Work out the finished part from the listing and answer in its coordinate system (mm). Give positions to 0.01 mm unless a question says otherwise; leave off trailing zeros. Loops run counter-clockwise (first coordinate to the right, second up) from the corner with the lowest first, then second, coordinate; pieces in that order, holes last. Notation, with made-up numbers: (69, 65.25) - (88, 65.25) arc R31 ccw to (88, 103.25) - close; hole circle Ø8 at (78, -11.75). An arc over 180 degrees is marked (long way). One line per question, with ' | ' between items. Start each with the question number.
1. Section C-C (z = -93.6) is taken. Determine the outline of the cut face in (x, y), plus the area to 3 significant figures.
2. Section D-D (x = -75) is taken. Determine the outline of the cut face in (y, z).
3. Find the intervals of material crossed by line 1 (X direction, y = 4, z = 74); line 2 (X direction, y = 3, z = -79.85) (3 decimals); line 3 (X direction, y = 3.25, z = -65), in increasing order.
4. This flat-tipped pin is pushed along its axis until it touches: pin 1 (4 mm diameter, centred on x = -15.59, z = 74, fed in from +Y) (3 decimals). Where does it stop, or does it pass through?
5. For a pull along X with two mould halves and no side action, classify faces 1 (the face through (32.2, 3.22, -81.83)), 2 (the face through (-1, 6.35, -1)) as released by +X, released by -X, zero draft, split by the parting line, or undercut.
6. Section B-B (x = 0) is taken. Determine the outline of the cut face in (y, z).
7. Section A-A (z = 65) is taken. Determine the outline of the cut face in (x, y).
from build123d import *

# Parameters (mm, degrees)
ESQUISSE1_W             = 203.2
ESQUISSE1_H             = 203.2
BOSS_EXTRU_1_DEPTH      = 6.35
ESQUISSE2_R             = 4
ENL_V_MAT_EXTRU_1_DEPTH = 144.824345992
ENL_V_MAT_EXTRU_2_DEPTH = 144.824345992
ESQUISSE5_R             = 2.5
ENL_V_MAT_EXTRU_4_DEPTH = 144.824345992
ESQUISSE6_R             = 2.5
ENL_V_MAT_EXTRU_5_DEPTH = 144.824345992
ESQUISSE7_R             = 2.5
ENL_V_MAT_EXTRU_6_DEPTH = 144.824345992


with BuildPart() as part:
    # Esquisse1 → Boss.-Extru.1 (new body)
    with BuildSketch(Plane(origin=(0, 0, 0), x_dir=(1, 0, 0), z_dir=(0, 1, 0))):
        Rectangle(ESQUISSE1_W, ESQUISSE1_H)
    extrude(amount=BOSS_EXTRU_1_DEPTH)

    # Esquisse2 → Enlèv. mat.-Extru.1 (cut, through all)
    with BuildSketch(Plane(origin=(0, 6.35, 0), x_dir=(1, 0, 0), z_dir=(0, 1, 0))):
        with Locations(Location((-75, 65, 0), (0, 0, 270))):
            Circle(ESQUISSE2_R)
        with Locations(Location((75, 65, 0), (0, 0, 270))):
            Circle(ESQUISSE2_R)
        with Locations(Location((0, -65, 0), (0, 0, 270))):
            Circle(ESQUISSE2_R)
    extrude(amount=-ENL_V_MAT_EXTRU_1_DEPTH, mode=Mode.SUBTRACT)

    # Esquisse3 → Enlèv. mat.-Extru.2 (cut, through all)
    with BuildSketch(Plane(origin=(0, 6.35, 0), x_dir=(1, 0, 0), z_dir=(0, 1, 0))):
        Polygon((-17.05, 86.15), (-21.15, 82.05), (-21.15, 47.95), (-17.05, 43.85), (17.05, 43.85), (21.15, 47.95), (21.15, 82.05), (17.05, 86.15), align=None)
    extrude(amount=-ENL_V_MAT_EXTRU_2_DEPTH, mode=Mode.SUBTRACT)

    # Esquisse5 → Enlèv. mat.-Extru.4 (cut, through all)
    with BuildSketch(Plane(origin=(0, 6.35, 0), x_dir=(1, 0, 0), z_dir=(0, 1, 0))):
        with Locations(Location((-33.425, 49.85, 0), (0, 0, 270))):
            Circle(ESQUISSE5_R)
        with Locations(Location((-33.425, 79.85, 0), (0, 0, 270))):
            Circle(ESQUISSE5_R)
        with Locations(Location((33.725, 49.85, 0), (0, 0, 270))):
            Circle(ESQUISSE5_R)
        with Locations(Location((33.725, 79.85, 0), (0, 0, 270))):
            Circle(ESQUISSE5_R)
    extrude(amount=-ENL_V_MAT_EXTRU_4_DEPTH, mode=Mode.SUBTRACT)

    # Esquisse6 → Enlèv. mat.-Extru.5 (cut, through all)
    with BuildSketch(Plane(origin=(0, 6.35, 0), x_dir=(1, 0, 0), z_dir=(0, 1, 0))):
        with Locations(Location((93.6, -93.6, 0), (0, 0, 270))):
            Circle(ESQUISSE6_R)
        with Locations(Location((-93.6, -93.6, 0), (0, 0, 270))):
            Circle(ESQUISSE6_R)
        with Locations(Location((-93.6, 93.6, 0), (0, 0, 270))):
            Circle(ESQUISSE6_R)
        with Locations(Location((93.6, 93.6, 0), (0, 0, 270))):
            Circle(ESQUISSE6_R)
    extrude(amount=-ENL_V_MAT_EXTRU_5_DEPTH, mode=Mode.SUBTRACT)

    # Esquisse7 → Enlèv. mat.-Extru.6 (cut, through all)
    with BuildSketch(Plane(origin=(0, 6.35, 0), x_dir=(1, 0, 0), z_dir=(0, 1, 0))):
        with Locations(Location((-15.588457268, -74, 0), (0, 0, 270))):
            Circle(ESQUISSE7_R)
        with Locations(Location((15.588457268, -74, 0), (0, 0, 270))):
            Circle(ESQUISSE7_R)
        with Locations(Location((0, -47, 0), (0, 0, 270))):
            Circle(ESQUISSE7_R)
        with Locations(Location((90.588457268, 56, 0), (0, 0, 270))):
            Circle(ESQUISSE7_R)
        with Locations(Location((59.411542732, 56, 0), (0, 0, 270))):
            Circle(ESQUISSE7_R)
        with Locations(Location((75, 83, 0), (0, 0, 270))):
            Circle(ESQUISSE7_R)
        with Locations(Location((-90.588457268, 56, 0), (0, 0, 270))):
            Circle(ESQUISSE7_R)
        with Locations(Location((-59.411542732, 56, 0), (0, 0, 270))):
            Circle(ESQUISSE7_R)
        with Locations(Location((-75, 83, 0), (0, 0, 270))):
            Circle(ESQUISSE7_R)
    extrude(amount=-ENL_V_MAT_EXTRU_6_DEPTH, mode=Mode.SUBTRACT)


solid = part.part
Conclusion:
1) outline: (-101.6, 0) - (-96.1, 0) - (-96.1, 6.35) - (-101.6, 6.35) - close; (-91.1, 0) - (91.1, 0) - (91.1, 6.35) - (-91.1, 6.35) - close; (96.1, 0) - (101.6, 0) - (101.6, 6.35) - (96.1, 6.35) - close | area: 1,230 mm²
2) outline: (0, -101.6) - (6.35, -101.6) - (6.35, -85.5) - (0, -85.5) - close; (0, -80.5) - (6.35, -80.5) - (6.35, -69) - (0, -69) - close; (0, -61) - (6.35, -61) - (6.35, 101.6) - (0, 101.6) - close
3) line 1: -101.6 to -18.09, -13.09 to 13.09, 18.09 to 101.6 | line 2: -101.6 to -35.925, -30.925 to -21.15, 21.15 to 31.225, 36.225 to 101.6 | line 3: -101.6 to -79, -71 to -21.15, 21.15 to 71, 79 to 101.6
4) pin 1: through
5) face 1: undercut | face 2: zero draft
6) outline: (0, -101.6) - (6.35, -101.6) - (6.35, -86.15) - (0, -86.15) - close; (0, -43.85) - (6.35, -43.85) - (6.35, 44.5) - (0, 44.5) - close; (0, 49.5) - (6.35, 49.5) - (6.35, 61) - (0, 61) - close; (0, 69) - (6.35, 69) - (6.35, 101.6) - (0, 101.6) - close
7) outline: (-101.6, 0) - (-4, 0) - (-4, 6.35) - (-101.6, 6.35) - close; (4, 0) - (101.6, 0) - (101.6, 6.35) - (4, 6.35) - close
